from build123d import *

# Parameters (mm, degrees)
BOSS_EXTRUDE1_DEPTH              = 330.2
BOSS_EXTRUDE1_DEPTH_BACK         = 330.2
SKETCH3_W                        = 50.8
SKETCH3_H                        = 25.4
SKETCH3_W_2                      = 44.45
SKETCH3_H_2                      = 19.05
F_1_4_0_25_DIAMETER_HOLE3_D      = 6.35
F_1_4_0_25_DIAMETER_HOLE4_D      = 6.35
F_1_4_0_25_DIAMETER_HOLE5_D      = 6.35
F_1_4_0_25_DIAMETER_HOLE6_D      = 6.35
F_1_4_0_25_DIAMETER_HOLE7_D      = 6.35
F_1_4_0_25_DIAMETER_HOLE8_D      = 6.35
F_13_64_0_20313_DIAMETER_HOLE1_D = 5.159502
F_1_2_0_5_DIAMETER_HOLE1_D       = 12.7
F_1_2_0_5_DIAMETER_HOLE1_DEPTH   = 6.35
F_1_2_0_5_DIAMETER_HOLE1_TIP     = 3.815464931
F_10_CLEARANCE_HOLE1_D           = 4.9784
F_10_CLEARANCE_HOLE1_DEPTH       = 25.4
F_10_CLEARANCE_HOLE1_TIP         = 1.495662253


with BuildPart() as part:
    # Sketch3 → Boss-Extrude1 (new, two sides: drawn at the far end of the back side and taken through both)
    with BuildSketch(Plane.XY.offset(-BOSS_EXTRUDE1_DEPTH_BACK)):
        Rectangle(SKETCH3_W, SKETCH3_H)
        Rectangle(SKETCH3_W_2, SKETCH3_H_2, mode=Mode.SUBTRACT)
    extrude(amount=BOSS_EXTRUDE1_DEPTH + BOSS_EXTRUDE1_DEPTH_BACK)

    # 1/4 (0.25) Diameter Hole3 (through all)
    with Locations(Plane.ZY.offset(25.4)):
        with Locations((-317.5, 0)):
            Hole(F_1_4_0_25_DIAMETER_HOLE3_D / 2)

    # 1/4 (0.25) Diameter Hole4 (through all)
    with Locations(Plane.ZY.offset(25.4)):
        with Locations((292.1, 0), (317.5, 0)):
            Hole(F_1_4_0_25_DIAMETER_HOLE4_D / 2)

    # 1/4 (0.25) Diameter Hole5 (through all)
    with Locations(Plane(origin=(25.4, 0, 0), x_dir=(0, 0, -1), z_dir=(1, 0, 0))):
        with Locations((292.1, 0), (266.7, 0)):
            Hole(F_1_4_0_25_DIAMETER_HOLE5_D / 2)

    # 1/4 (0.25) Diameter Hole6 (through all)
    with Locations(Plane(origin=(25.4, 0, 0), x_dir=(0, 0, -1), z_dir=(1, 0, 0))):
        with Locations((215.9, 0), (241.3, 0)):
            Hole(F_1_4_0_25_DIAMETER_HOLE6_D / 2)

    # 1/4 (0.25) Diameter Hole7 (through all)
    with Locations(Plane(origin=(25.4, 0, 0), x_dir=(0, 0, -1), z_dir=(1, 0, 0))):
        with Locations((-190.5, 0), (-215.9, 0)):
            Hole(F_1_4_0_25_DIAMETER_HOLE7_D / 2)

    # 1/4 (0.25) Diameter Hole8 (through all)
    with Locations(Plane(origin=(25.4, 0, 0), x_dir=(0, 0, -1), z_dir=(1, 0, 0))):
        with Locations((-266.7, 0), (-241.3, 0)):
            Hole(F_1_4_0_25_DIAMETER_HOLE8_D / 2)

    # 13/64 (0.20313) Diameter Hole1 (through all)
    with Locations(Plane(origin=(25.4, 0, 0), x_dir=(0, 0, -1), z_dir=(1, 0, 0))):
        with Locations((-152.4, 0), (177.8, 0)):
            Hole(F_13_64_0_20313_DIAMETER_HOLE1_D / 2)

    # 1/2 (0.5) Diameter Hole1
    with Locations(Plane.ZY.offset(25.4)):
        with Locations((-146.050000508, 4.9e-08), (120.65, 1.7e-08)):
            Hole(F_1_2_0_5_DIAMETER_HOLE1_D / 2, depth=F_1_2_0_5_DIAMETER_HOLE1_DEPTH)
            with Locations((0, 0, -(F_1_2_0_5_DIAMETER_HOLE1_DEPTH + F_1_2_0_5_DIAMETER_HOLE1_TIP / 2))):  # 118° drill point
                Cone(0, F_1_2_0_5_DIAMETER_HOLE1_D / 2, F_1_2_0_5_DIAMETER_HOLE1_TIP, mode=Mode.SUBTRACT)

    # #10 Clearance Hole1
    with Locations(Plane(origin=(0, -12.7, 0), x_dir=(-1, 0, 0), z_dir=(0, -1, 0))):
        with Locations((7.747762, 30.0312328), (-17.652238, 30.0312328), (-17.652238, -128.7187672), (7.747762, -128.7187672)):
            Hole(F_10_CLEARANCE_HOLE1_D / 2, depth=F_10_CLEARANCE_HOLE1_DEPTH)
            with Locations((0, 0, -(F_10_CLEARANCE_HOLE1_DEPTH + F_10_CLEARANCE_HOLE1_TIP / 2))):  # 118° drill point
                Cone(0, F_10_CLEARANCE_HOLE1_D / 2, F_10_CLEARANCE_HOLE1_TIP, mode=Mode.SUBTRACT)


solid = part.part
CAD build for the part. Positions are in the model's coordinates, mm. A direction names the side the tool comes from. Round coordinates to 2 decimals unless told otherwise and drop trailing zeros. Write each loop counter-clockwise with the first axis right and the second up, starting at its lowest first coordinate (ties: lowest second). Pieces come first, ordered by that corner, then holes.
(1) 3-axis set-ups, long thin cutter, end or side, ignore diameter. For faces 5 (the face through (-23.79, 1.907, -152.107)), 6 (the face through (0, -12.7, -5)), 7 (the face through (22.225, 0, -5)): which of +Z, -Z, +X, -X, +Y, -Y reach the whole face in a straight line?
(2) Slice it at A-A, the plane z = 276. Write the cut outline in (x, y) (3 decimals), and give its area (3 significant figures).
(3) Slice it at C-C, the plane z = 120.65. Write the cut outline in (x, y) (3 decimals).
(4) Slice it at B-B, the plane x = 0.5. Write the cut outline in (y, z) (3 decimals), and give its area (3 significant figures).
(5) Probe line 1 along Z through (x, y) = (18, -10.25); line 2 along Y through (x, z) = (-23.05, 266.7) (3 decimals); line 3 along Y through (x, z) = (7, -189.5) (3 decimals). List the from-to ranges inside material, lowest first.
(6) Mould opens along X. For faces 1 (the face through (0, -9.525, -5)), 2 (the face through (0, 10, -330.2)), 3 (the face through (25.4, 0, -5)), 4 (the face through (0, 9.525, -5)) say: pulls with the +X half, pulls with the -X half, needs draft (parallel to the pull), parting line crosses it, or undercut.
From the geometry:
1. face 5: -X
1. face 6: +Z, -Z, +X, -X, -Y
1. face 7: +Z, -Z
2. outline: (-25.4, -12.7) - (25.4, -12.7) - (25.4, 12.7) - (-25.4, 12.7) - close; hole (-22.225, -9.525) - (22.225, -9.525) - (22.225, 9.525) - (-22.225, 9.525) - close
2. area: 444 mm2
3. outline: (-25.4, -12.7) - (25.4, -12.7) - (25.4, 12.7) - (-25.4, 12.7) - (-25.4, 6.35) - (-22.225, 6.35) - (-22.225, 9.525) - (22.225, 9.525) - (22.225, -9.525) - (-22.225, -9.525) - (-22.225, -6.35) - (-25.4, -6.35) - close
4. outline: (-12.7, -330.2) - (-9.525, -330.2) - (-9.525, 330.2) - (-12.7, 330.2) - close; (9.525, -330.2) - (12.7, -330.2) - (12.7, 330.2) - (9.525, 330.2) - close
4. area: 4,190 mm2
5. line 1: z = -330.2 to -32.5, -27.57 to 126.25, 131.18 to 330.2
5. line 2: y = -12.7 to -3.175, 3.175 to 12.7
5. line 3: y = -12.7 to -9.525, 9.525 to 12.7
6. face 1: undercut
6. face 2: needs draft
6. face 3: pulls with the +X half
6. face 4: undercut
